The drawing under review shows one solid part. Ordinate dimensions are in mm from its lowest x, y, z. A direction names the side the tool comes from. Coordinates: 2 decimals unless noted, no trailing zeros. Write each loop counter-clockwise with the first axis right and the second up, starting at its lowest first coordinate (ties: lowest second). Pieces come first, ordered by that corner, then holes.
1) For P1, Ø10, axis at y = 84, z = 5, coming from the -X side; P2, Ø1, axis at x = 16, y = 56.5, coming from the -Z side; P3, Ø8, axis at y = 114, z = 3.5, coming from the -X side, all flat-tipped, find the tip position at first contact; note any pin that passes through.
2) For line 1 (Y direction, x = 15, z = 21); line 2 (X direction, y = 145.5, z = 13.5); line 3 (Y direction, x = 22.75, z = 17.25), list the stretches that pass through material, from the lowest coordinate up.
3) Add section D-D, the plane y = 25. State the section outline as (x, z) points.
4) Add section B-B, the plane z = 13.5. State the section outline as (x, y) points.
5) Add section C-C, the plane y = 88. State the section outline as (x, z) points.
6) Add section A-A, the plane x = 13.5. State the section outline as (y, z) points.
7) Machinability: for the marked faces 1, 2 and 3, which of the approach directions +Z, -Z, +X, -X, +Y, -Y give a long, thin tool a straight path to every point of the face, cutting with its end or side? Answer none if there is none.
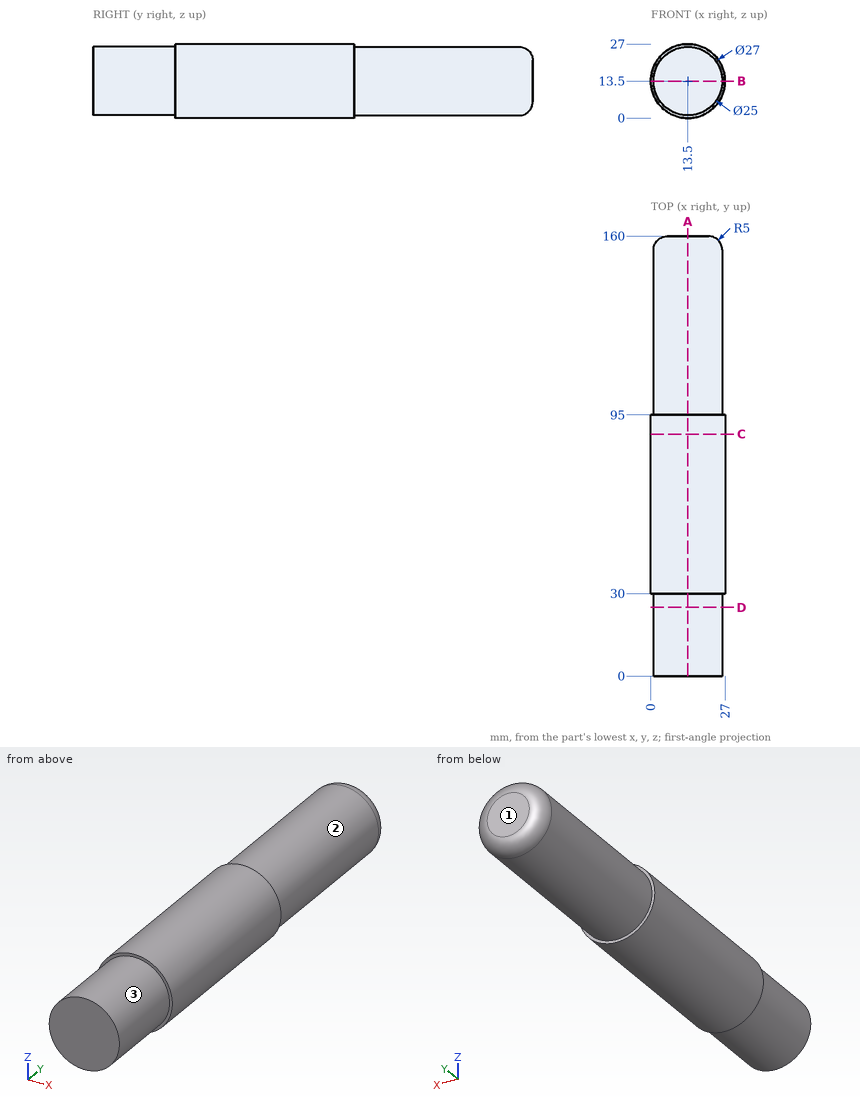
Geometry results:
1. P1: stops at x = 0.46
1. P2: stops at z = 0.15
1. P3: stops at x = 2.53
2. line 1: y = 0 to 160
2. line 2: x = 1 to 26
2. line 3: y = 0 to 159.34
3. outline: circle Ø25 at (13.5, 13.5)
4. outline: (0, 30) - (1, 30) - (1, 0) - (26, 0) - (26, 30) - (27, 30) - (27, 95) - (26, 95) - (26, 155) arc R5 ccw to (21, 160) - (6, 160) arc R5 ccw to (1, 155) - (1, 95) - (0, 95) - close
5. outline: circle Ø27 at (13.5, 13.5)
6. outline: (0, 1) - (30, 1) - (30, 0) - (95, 0) - (95, 1) - (155, 1) arc R5 ccw to (160, 6) - (160, 21) arc R5 ccw to (155, 26) - (95, 26) - (95, 27) - (30, 27) - (30, 26) - (0, 26) - close
7. face 1: +Z, -Z, +X, -X, +Y
7. face 2: +Y
7. face 3: -Y
